For this review, take the finished solid that the model builds, in its own axes (mm). A direction names the side the tool comes from. Round coordinates to 2 decimals unless told otherwise and drop trailing zeros. Order: outer loops, then holes, each group sorted by start corner. A loop starts at its lowest first (then second) coordinate and runs counter-clockwise, first axis right, second up. Notation, with made-up numbers: M 26,53 L 41,53 A15 cw 41,67 Z; hole C 26.25,20 d2. An arc over 180 degrees is marked long. Put each result on its own line as item: value.
from build123d import *

# Parameters (mm, degrees)
SKETCH1_W                 = 25.4
SKETCH1_H                 = 50.8
SKETCH1_W_2               = 19.05
SKETCH1_H_2               = 44.45
BOSS_EXTRUDE1_DEPTH       = 199.62495
F_8_32_TAPPED_HOLE1_D     = 3.4544
F_8_32_TAPPED_HOLE1_DEPTH = 3.175
CUT_EXTRUDE2_DEPTH        = 203.831064343
FILLET1_R                 = 3.175
F_8_32_TAPPED_HOLE2_D     = 3.4544
F_8_32_TAPPED_HOLE2_DEPTH = 3.175
F_8_32_TAPPED_HOLE3_D     = 3.4544
F_8_32_TAPPED_HOLE3_DEPTH = 3.175


with BuildPart() as part:
    # Sketch1 → Boss-Extrude1 (new, symmetric)
    with BuildSketch(Plane(origin=(0, 0, 0), x_dir=(0, 0, -1), z_dir=(1, 0, 0))):
        Rectangle(SKETCH1_W, SKETCH1_H)
        Rectangle(SKETCH1_W_2, SKETCH1_H_2, mode=Mode.SUBTRACT)
    extrude(amount=BOSS_EXTRUDE1_DEPTH, both=True)

    # #8-32 Tapped Hole1
    with Locations(Plane.XY.offset(12.7)):
        with Locations((166.28745, 19.05), (166.28745, -19.05), (-166.28745, 19.05), (-166.28745, -19.05)):
            Hole(F_8_32_TAPPED_HOLE1_D / 2, depth=F_8_32_TAPPED_HOLE1_DEPTH)

    # Sketch5 → Cut-Extrude2 (cut, through all)
    with BuildSketch(Plane.XY.offset(12.7)):
        Polygon((-153.58745, 19.05), (-153.58745, -13.113403304), (-110.368770238, 19.05), align=None)
        Polygon((-145.610313096, -19.05), (-102.391633333, 13.113403304), (-59.172953571, -19.05), align=None)
        Polygon((-94.414496429, 19.05), (-7.977136904, 19.05), (-51.195816667, -13.113403304), align=None)
        Polygon((-43.218679762, -19.05), (0, 13.113403304), (43.218679762, -19.05), align=None)
        Polygon((94.414496429, 19.05), (51.195816667, -13.113403304), (7.977136904, 19.05), align=None)
        Polygon((59.172953571, -19.05), (102.391633333, 13.113403304), (145.610313096, -19.05), align=None)
        Polygon((110.368770238, 19.05), (153.58745, 19.05), (153.58745, -13.113403304), align=None)
    extrude(amount=-CUT_EXTRUDE2_DEPTH, mode=Mode.SUBTRACT)

    # Fillet1
    fillet1_edges = [part.edges().sort_by_distance(p)[0] for p in [
        (-94.414496429, 19.05, 11.1125),
        (-7.977136904, 19.05, 11.1125),
        (43.218679762, -19.05, -11.1125),
        (-43.218679762, -19.05, -11.1125),
        (0, 13.113403304, -11.1125),
        (43.218679762, -19.05, 11.1125),
        (-43.218679762, -19.05, 11.1125),
        (0, 13.113403304, 11.1125),
        (7.977136904, 19.05, -11.1125),
        (94.414496429, 19.05, -11.1125),
        (51.195816667, -13.113403304, -11.1125),
        (7.977136904, 19.05, 11.1125),
        (94.414496429, 19.05, 11.1125),
        (51.195816667, -13.113403304, 11.1125),
        (145.610313096, -19.05, -11.1125),
        (59.172953571, -19.05, -11.1125),
        (102.391633333, 13.113403304, -11.1125),
        (145.610313096, -19.05, 11.1125),
        (59.172953571, -19.05, 11.1125),
        (102.391633333, 13.113403304, 11.1125),
        (153.58745, -13.113403304, -11.1125),
        (110.368770238, 19.05, -11.1125),
        (153.58745, 19.05, -11.1125),
        (153.58745, -13.113403304, 11.1125),
        (110.368770238, 19.05, 11.1125),
        (153.58745, 19.05, 11.1125),
        (-153.58745, 19.05, -11.1125),
        (-110.368770238, 19.05, -11.1125),
        (-153.58745, -13.113403304, -11.1125),
        (-153.58745, 19.05, 11.1125),
        (-110.368770238, 19.05, 11.1125),
        (-153.58745, -13.113403304, 11.1125),
        (-59.172953571, -19.05, -11.1125),
        (-145.610313096, -19.05, -11.1125),
        (-102.391633333, 13.113403304, -11.1125),
        (-59.172953571, -19.05, 11.1125),
        (-145.610313096, -19.05, 11.1125),
        (-102.391633333, 13.113403304, 11.1125),
        (-51.195816667, -13.113403304, -11.1125),
        (-94.414496429, 19.05, -11.1125),
        (-7.977136904, 19.05, -11.1125),
        (-51.195816667, -13.113403304, 11.1125),
    ]]
    fillet(fillet1_edges, radius=FILLET1_R)

    # #8-32 Tapped Hole2
    with Locations(Plane(origin=(0, 0, -12.7), x_dir=(-1, 0, 0), z_dir=(0, 0, -1))):
        with Locations((-183.74995, 19.05), (-183.74995, -19.05), (183.74995, -19.05), (183.74995, 19.05)):
            Hole(F_8_32_TAPPED_HOLE2_D / 2, depth=F_8_32_TAPPED_HOLE2_DEPTH)

    # #8-32 Tapped Hole3
    with Locations(Plane(origin=(0, 25.4, 0), x_dir=(1, 0, 0), z_dir=(0, 1, 0))):
        with Locations((-152.4, -0.27178), (-50.8, -0.27178), (50.8, -0.27178), (152.4, -0.27178)):
            Hole(F_8_32_TAPPED_HOLE3_D / 2, depth=F_8_32_TAPPED_HOLE3_DEPTH)


solid = part.part
(1) To check wall thickness, follow L1, parallel to Z at x = -152, y = 24; L2, parallel to Z at x = -76, y = 4.5 (3 decimals); L3, parallel to Y at x = 121.5, z = -8.5 (3 decimals). State the ranges of each line that lie inside material, in increasing order.
A:
L1: z = -12.7 to -1.41, 1.95 to 12.7
L2: z = -12.7 to -9.525, 9.525 to 12.7
L3: y = -25.4 to -22.225, 22.225 to 25.4
(2) Add section B-B on x = -6.5. Give the boundary of the cut face in (y, z) (3 decimals).
A:
outline: M -25.4,-12.7 L -19.05,-12.7 L -19.05,-9.525 L -22.225,-9.525 L -22.225,9.525 L -19.05,9.525 L -19.05,12.7 L -25.4,12.7 Z; M 8.276,-12.7 L 25.4,-12.7 L 25.4,12.7 L 8.276,12.7 L 8.276,9.525 L 22.225,9.525 L 22.225,-9.525 L 8.276,-9.525 Z
(3) Insertion check: pin 1 Ø5 at (y, z) = (-17.5, 6) entering from -X. The pin has a flat end and moves straight along its axis. Give the tip position at first contact, or say it passes through.
A:
pin 1: passes through
(4) For faces 1 (the face through (3, 22.225, 0)), 2 (the face through (3, 17, -12.7)), 3 (the face through (-83.91, -0.64, -11.09)), list the 3-axis set-ups (+Z, -Z, +X, -X, +Y, -Y) from which the entire face can be reached by the end or side of a thin tool; tool diameter is ignored.
A:
face 1: +X, -X
face 2: -Z, +X, -X, +Y, -Y
face 3: +Z, -Z
(5) Draft analysis for pull direction X (two halves, no side actions). For faces 4 (the face through (199.625, -2, 10)), 5 (the face through (3, 15, -9.525)), 6 (the face through (-133.5, 1.835, 11.135)), state which applies: released by +X, released by -X, zero draft, split by the parting line, or undercut.
A:
face 4: released by +X
face 5: zero draft
face 6: undercut
(6) Add section A-A on x = 125. Give the boundary of the cut face in (y, z) (3 decimals), then the cut area to 3 significant figures.
A:
outline: M -25.4,-12.7 L -19.05,-12.7 L -19.05,-9.525 L -22.225,-9.525 L -22.225,9.525 L -19.05,9.525 L -19.05,12.7 L -25.4,12.7 Z; M -3.712,-12.7 L 8.161,-12.7 L 8.161,-9.525 L -3.712,-9.525 Z; M -3.712,9.525 L 8.161,9.525 L 8.161,12.7 L -3.712,12.7 Z; M 19.05,-12.7 L 25.4,-12.7 L 25.4,12.7 L 19.05,12.7 L 19.05,9.525 L 22.225,9.525 L 22.225,-9.525 L 19.05,-9.525 Z
area: 277 mm2
(7) Add section C-C on x = -159. Give the boundary of the cut face in (y, z) (3 decimals), then the cut area to 3 significant figures.
A:
outline: M -25.4,-12.7 L 25.4,-12.7 L 25.4,12.7 L -25.4,12.7 Z; hole M -22.225,-9.525 L 22.225,-9.525 L 22.225,9.525 L -22.225,9.525 Z
area: 444 mm2
